Check sheet for the modelled part. Datum: model origin and axes. Units: mm. A direction names the side the tool comes from. Coordinates: 2 decimals unless noted, no trailing zeros. Order: outer loops, then holes, each group sorted by start corner. A loop starts at its lowest first (then second) coordinate and runs counter-clockwise, first axis right, second up.
from build123d import *

# Parameters (mm, degrees)
SKETCH_1_R          = 4.5
EXTRUDE_2_DEPTH     = 4
CUT_EXTRUDE_1_DEPTH = 83.559069762
FILLET_1_R          = 3
SKETCH_6_R          = 1.7
CUT_EXTRUDE_2_DEPTH = 83.559069762
SKETCH_7_R          = 8.75
CUT_EXTRUDE_3_DEPTH = 1.5


with BuildPart() as part:
    # 草图1 → 凸台-拉伸2 (new body)
    with BuildSketch(Plane.XY):
        with BuildLine():
            Line((20, -60), (20, 60))
            ThreePointArc((20, 60), (0, 80), (-20, 60))
            Line((-20, 60), (-20, -60))
            ThreePointArc((-20, -60), (0, -80), (20, -60))
        make_face()
        with Locations((0, 60)):
            Circle(SKETCH_1_R, mode=Mode.SUBTRACT)
        with Locations((0, -60)):
            Circle(SKETCH_1_R, mode=Mode.SUBTRACT)
    extrude(amount=EXTRUDE_2_DEPTH)

    # 草图4 → 切除-拉伸1 (cut, through all)
    with BuildSketch(Plane.XY.offset(4)):
        Polygon((-14, -18.844505579), (11.137802231, 44), (-14, 44), align=None)
        Polygon((14, -44), (14, 18.844505579), (-11.137802231, -44), align=None)
    extrude(amount=-CUT_EXTRUDE_1_DEPTH, mode=Mode.SUBTRACT)

    # 圆角1
    fillet_1_edges = [part.edges().sort_by_distance(p)[0] for p in [
        (14, -44, 2),
        (-11.137802231, -44, 2),
        (14, 18.844505579, 2),
        (-14, -18.844505579, 2),
        (-14, 44, 2),
        (11.137802231, 44, 2),
    ]]
    fillet(fillet_1_edges, radius=FILLET_1_R)

    # 草图6 → 切除-拉伸2 (cut, through all)
    with BuildSketch(Plane.XY.offset(4)):
        with Locations((0, 50)):
            Circle(SKETCH_6_R)
        with Locations((-8.660254038, 55)):
            Circle(SKETCH_6_R)
        with Locations((-8.660254038, 65)):
            Circle(SKETCH_6_R)
        with Locations((0, 70)):
            Circle(SKETCH_6_R)
        with Locations((8.660254038, 65)):
            Circle(SKETCH_6_R)
        with Locations((8.660254038, 55)):
            Circle(SKETCH_6_R)
    extrude(amount=-CUT_EXTRUDE_2_DEPTH, mode=Mode.SUBTRACT)

    # 草图7 → 切除-拉伸3 (cut)
    with BuildSketch(Plane.XY.offset(4)):
        with Locations((0, -60)):
            Circle(SKETCH_7_R)
    extrude(amount=-CUT_EXTRUDE_3_DEPTH, mode=Mode.SUBTRACT)


solid = part.part
(1) Release check for a two-part mould opening along Y. For faces 3 (the flat face through (-2, 44, 2)), 4 (the cylindrical face through (0, -80, 2)), 5 (the cylindrical face through (0, 80, 2)) record: +Y half, -Y half, draft (parallel to the pull), parting line (faces both ways), or undercut.
Filled in:
face 3: undercut
face 4: -Y half
face 5: +Y half
(2) Cross-section at B-B (y = -8.5). Enter the section's corners in (x, z).
Filled in:
outline: (-20, 0) - (3.06, 0) - (3.06, 4) - (-20, 4) - close; (14, 0) - (20, 0) - (20, 4) - (14, 4) - close
(3) Tool access check on faces 1 (the flat face through (14, -19, 2)), 2 (the flat face through (-20, 1, 2)). Record the directions out of +Z, -Z, +X, -X, +Y, -Y that give a thin tool (end or side, any length) a straight path to the whole face; none if there is none.
Filled in:
face 1: +Z, -Z
face 2: +Z, -Z, -X, +Y, -Y
(4) Thickness scan on probe 1 along X at (y, z) = (38, 2.55); probe 2 along X at (y, z) = (65, 1); probe 3 along X at (y, z) = (39.5, 2.6). Record the ranges inside material, lowest first.
Filled in:
probe 1: x = -20 to -14, 8.74 to 20
probe 2: x = -19.36 to -10.36, -6.96 to 6.96, 10.36 to 19.36
probe 3: x = -20 to -14, 9.34 to 20
(5) Go/stop test with flat-tipped pins: P1, Ø2, axis at x = -2, z = 2, coming from the +Y side (3 decimals); P2, Ø2, axis at x = -11, z = 3, coming from the -Y side; P3, Ø14.5, axis at x = 0, y = -60, coming from the +Z side. Record where each tip stops, or that it passes through.
Filled in:
P1: stops at y = 79.975
P2: stops at y = -77.32
P3: stops at z = 2.5
(6) Cross-section at D-D (y = -30.5). Enter the section's corners in (x, z).
Filled in:
outline: (-20, 0) - (-5.74, 0) - (-5.74, 4) - (-20, 4) - close; (14, 0) - (20, 0) - (20, 4) - (14, 4) - close
(7) Cross-section at A-A (z = 1.8). Count the separate pieces of the cut face and the enclosed holes in it, and give its area (3 significant figures).
Filled in:
separate pieces: 1
enclosed holes: 10
area: 4,380 mm2
